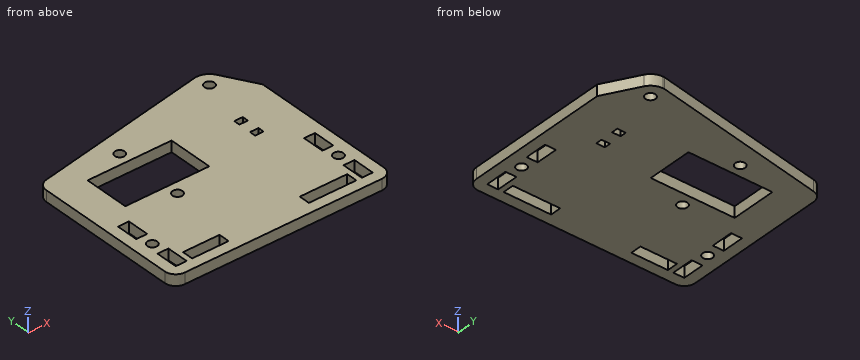
from build123d import *

# Parameters (mm, degrees)
SKETCH_1_R      = 1.359
SKETCH_1_W      = 2.329
SKETCH_1_H      = 1.693
SKETCH_1_W_2    = 12.999
SKETCH_1_H_2    = 3
SKETCH_1_W_3    = 10
SKETCH_1_W_4    = 3
SKETCH_1_H_3    = 6.001
SKETCH_1_W_5    = 23
SKETCH_1_H_4    = 12.399
EXTRUDE_1_DEPTH = 3


with BuildPart() as part:
    # 草图1 → 凸台-拉伸1 (new body)
    with BuildSketch(Plane.XY.offset(3)):
        with BuildLine():
            Line((3, -27.964431369), (57, -27.964431369))
            ThreePointArc((57, -27.964431369), (59.121320344, -27.085751712), (60, -24.964431369))
            Line((60, -24.964431369), (60, 14.844527968))
            Line((60, 14.844527968), (54.721484389, 23.930621486))
            ThreePointArc((54.721484389, 23.930621486), (53.258114674, 25.388095235), (51.262778196, 25.921305316))
            Line((51.262778196, 25.921305316), (50.782638999, 25.921305316))
            Line((50.782638999, 25.921305316), (2.454554127, 16.985586191))
            ThreePointArc((2.454554127, 16.985586191), (0.693884476, 15.954397926), (0, 14.035588089))
            Line((0, 14.035588089), (0, -24.964431369))
            ThreePointArc((0, -24.964431369), (0.878679656, -27.085751712), (3, -27.964431369))
        make_face()
        with Locations(Location((51.251, 21.869668631, 0), (0, 0, 180))):
            Circle(SKETCH_1_R, mode=Mode.SUBTRACT)
        with Locations(Location((20.499, 14.465668631, 0), (0, 0, 180))):
            Circle(SKETCH_1_R, mode=Mode.SUBTRACT)
        with Locations(Location((20.499, -4.535331369, 0), (0, 0, 180))):
            Circle(SKETCH_1_R, mode=Mode.SUBTRACT)
        with Locations(Location((4.5, -15.464331369, 0), (0, 0, 180))):
            Circle(SKETCH_1_R, mode=Mode.SUBTRACT)
        with Locations(Location((55.5, -15.464331369, 0), (0, 0, 180))):
            Circle(SKETCH_1_R, mode=Mode.SUBTRACT)
        with Locations((47.8435, 2.205168631)):
            Rectangle(SKETCH_1_W, SKETCH_1_H, mode=Mode.SUBTRACT)
        with Locations((47.8955, 7.444168631)):
            Rectangle(SKETCH_1_W, SKETCH_1_H, mode=Mode.SUBTRACT)
        with Locations((45.9995, -23.464331369)):
            Rectangle(SKETCH_1_W_2, SKETCH_1_H_2, mode=Mode.SUBTRACT)
        with Locations((12.5, -23.464331369)):
            Rectangle(SKETCH_1_W_3, SKETCH_1_H_2, mode=Mode.SUBTRACT)
        with Locations((55.5, -8.964831369)):
            Rectangle(SKETCH_1_W_4, SKETCH_1_H_3, mode=Mode.SUBTRACT)
        with Locations((55.5, -21.963831369)):
            Rectangle(SKETCH_1_W_4, SKETCH_1_H_3, mode=Mode.SUBTRACT)
        with Locations((4.501, -21.963831369)):
            Rectangle(SKETCH_1_W_4, SKETCH_1_H_3, mode=Mode.SUBTRACT)
        with Locations((4.501, -8.964831369)):
            Rectangle(SKETCH_1_W_4, SKETCH_1_H_3, mode=Mode.SUBTRACT)
        with Locations((20.5, 5.035168631)):
            Rectangle(SKETCH_1_W_5, SKETCH_1_H_4, mode=Mode.SUBTRACT)
    extrude(amount=-EXTRUDE_1_DEPTH)


solid = part.part
Check sheet for the modelled part. Datum: model origin and axes. Units: mm. Give positions to 0.01 mm unless a question says otherwise; leave off trailing zeros. Write each loop counter-clockwise with the first axis right and the second up, starting at its lowest first coordinate (ties: lowest second). Pieces come first, ordered by that corner, then holes. Notation, with made-up numbers: (-9.75, 5.5) -> (44.25, 5.5) arc R11 ccw to (44.25, 19.5) -> close; hole circle Ø3 at (77, 38.5). An arc over 180 degrees is marked (long way). Write item = value, one per line.
Item 1: Sectioned sample at D-D on x = 4.5. Record the boundary of the cut face in (y, z).
Output:
outline = (-27.96, 0) -> (-24.96, 0) -> (-24.96, 3) -> (-27.96, 3) -> close; (-18.96, 0) -> (-16.82, 0) -> (-16.82, 3) -> (-18.96, 3) -> close; (-14.11, 0) -> (-11.97, 0) -> (-11.97, 3) -> (-14.11, 3) -> close; (-5.96, 0) -> (17.36, 0) -> (17.36, 3) -> (-5.96, 3) -> close
Item 2: Gauge pin test, flat ends, axial feed: pin 1 (1.5 mm diameter, centred on x = 31, z = 2, fed in from +Y); pin 2 (1.5 mm diameter, centred on x = 55.5, z = 1.5, fed in from +Y). Record the tip position at first contact, or that the pin passes through.
Output:
pin_1 = 22.4
pin_2 = 23.88
Item 3: Sectioned sample at A-A on y = -21. Record the boundary of the cut face in (x, z), and give its area (3 significant figures).
Output:
outline = (0, 0) -> (3, 0) -> (3, 3) -> (0, 3) -> close; (6, 0) -> (54, 0) -> (54, 3) -> (6, 3) -> close; (57, 0) -> (60, 0) -> (60, 3) -> (57, 3) -> close
area = 162 mm^2
Item 4: Sectioned sample at B-B on x = 30.5. Record the boundary of the cut face in (y, z), and give its area (3 significant figures).
Output:
outline = (-27.96, 0) -> (-1.16, 0) -> (-1.16, 3) -> (-27.96, 3) -> close; (11.23, 0) -> (22.17, 0) -> (22.17, 3) -> (11.23, 3) -> close
area = 113 mm^2
Item 5: Scan lines: probe 1 along X at (y, z) = (-23, 1.9); probe 2 along X at (y, z) = (5.5, 2.35); probe 3 along Y at (x, z) = (11.5, 1.4). Record each from-to range of solid material in increasing order. Write a range as from..to.
Output:
probe_1 = 0..3, 6..7.5, 17.5..39.5, 52.5..54, 57..60
probe_2 = 0..9, 32..60
probe_3 = -27.96..-24.96, -21.96..-1.16, 11.23..18.66
Item 6: Sectioned sample at C-C on x = 10.5. Record the boundary of the cut face in (y, z), and give its area (3 significant figures).
Output:
outline = (-27.96, 0) -> (-24.96, 0) -> (-24.96, 3) -> (-27.96, 3) -> close; (-21.96, 0) -> (-1.16, 0) -> (-1.16, 3) -> (-21.96, 3) -> close; (11.23, 0) -> (18.47, 0) -> (18.47, 3) -> (11.23, 3) -> close
area = 93.1 mm^2
